```python
from build123d import *

# Parameters (mm, degrees)
EXTRUDE_2_DEPTH          = 51
HOLE_WIZARD_M2_5_1_D     = 2.05
HOLE_WIZARD_M2_5_1_DEPTH = 4.75
HOLE_WIZARD_M2_5_1_TIP   = 0.615882135
SKETCH_7_R               = 11
SKETCH_7_R_2             = 2.5
EXTRUDE_3_DEPTH          = 2
SKETCH_7_2_R             = 2.5
EXTRUDE_4_DEPTH          = 20
SKETCH_8_W               = 15
SKETCH_8_H               = 0.5
CUT_EXTRUDE_1_DEPTH      = 1.5
SKETCH_9_W               = 15.5
SKETCH_9_H               = 2.6
EXTRUDE_5_DEPTH          = 6


with BuildPart() as part:
    # 草图1 → 凸台-拉伸2 (new body)
    with BuildSketch(Plane.XY):
        with BuildLine():
            Line((-12.1, -14.1), (12.1, -14.1))
            ThreePointArc((12.1, -14.1), (13.514213562, -13.514213562), (14.1, -12.1))
            Line((14.1, -12.1), (14.1, 12.1))
            ThreePointArc((14.1, 12.1), (13.514213562, 13.514213562), (12.1, 14.1))
            Line((12.1, 14.1), (-12.1, 14.1))
            ThreePointArc((-12.1, 14.1), (-13.514213562, 13.514213562), (-14.1, 12.1))
            Line((-14.1, 12.1), (-14.1, -12.1))
            ThreePointArc((-14.1, -12.1), (-13.514213562, -13.514213562), (-12.1, -14.1))
        make_face()
    extrude(amount=EXTRUDE_2_DEPTH)

    # M2.5 螺纹孔1
    with Locations(Plane(origin=(0, 0, 0), x_dir=(-1, 0, 0), z_dir=(0, 0, -1))):
        with Locations((-11.5, 11.5), (11.5, 11.5), (11.5, -11.5), (-11.5, -11.5)):
            Hole(HOLE_WIZARD_M2_5_1_D / 2, depth=HOLE_WIZARD_M2_5_1_DEPTH)
            with Locations((0, 0, -(HOLE_WIZARD_M2_5_1_DEPTH + HOLE_WIZARD_M2_5_1_TIP / 2))):  # 118° drill point
                Cone(0, HOLE_WIZARD_M2_5_1_D / 2, HOLE_WIZARD_M2_5_1_TIP, mode=Mode.SUBTRACT)

    # 草图7 → 凸台-拉伸3 (add)
    with BuildSketch(Plane.XY):
        Circle(SKETCH_7_R)
        Circle(SKETCH_7_R_2, mode=Mode.SUBTRACT)
    extrude(amount=-EXTRUDE_3_DEPTH)

    # 草图7<2> → 凸台-拉伸4 (add)
    with BuildSketch(Plane.XY):
        Circle(SKETCH_7_2_R)
    extrude(amount=-EXTRUDE_4_DEPTH)

    # 草图8 → 切除-拉伸1 (cut, symmetric)
    with BuildSketch(Plane(origin=(0, 0, 0), x_dir=(0, 0, -1), z_dir=(1, 0, 0))):
        with Locations((12.5, 2.25)):
            Rectangle(SKETCH_8_W, SKETCH_8_H)
    extrude(amount=CUT_EXTRUDE_1_DEPTH, both=True, mode=Mode.SUBTRACT)

    # 草图9 → 凸台-拉伸5 (add)
    with BuildSketch(Plane.XY.offset(44)):
        with Locations((0, -15.4)):
            Rectangle(SKETCH_9_W, SKETCH_9_H)
    extrude(amount=EXTRUDE_5_DEPTH)


solid = part.part
```
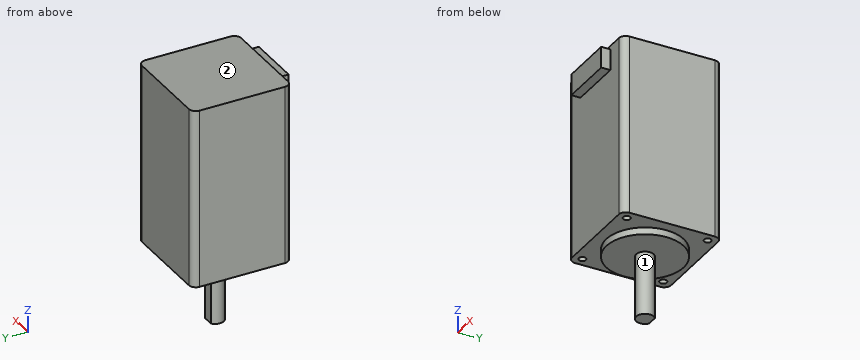
Geometry: final body of the model. Coordinates: model frame, mm. Face numbers are marked on the shaded views. A direction names the side the tool comes from. Coordinates: 2 decimals unless noted, no trailing zeros. Write each loop counter-clockwise with the first axis right and the second up, starting at its lowest first coordinate (ties: lowest second). Pieces come first, ordered by that corner, then holes. Notation, with made-up numbers: M -40,56 L -18,56 A24 ccw -18,90 Z; hole C 55,72 d7. An arc over 180 degrees is marked long. Answer as CSV lines item,"result". Start each with the question number.
Q1. Reachability of the marked faces 1 and 2 from +Z, -Z, +X, -X, +Y, -Y: full face, straight path, thin tool, end or side. Return the list, or none.
Q2. Cut plane B-B on y = 0. Return the cut outline in (x, z).
Q3. Pin query (flat end, axial travel): P1, Ø0.9, axis at x = -0.5, z = -10, coming from the +Y side; P2, Ø5, axis at x = 2.5, z = 14.5, coming from the -Y side; P3, Ø1.8, axis at x = 11.5, y = 11.5, coming from the -Z side. Return the tip coordinate at first contact, or that it passes through.
Q4. Cut plane A-A on z = 4. Return the cut outline in (x, y) (3 decimals).
Q5. Line query: line 1 (Y direction, x = -11.5, z = 2.7) (3 decimals); line 2 (X direction, y = -11, z = 3). Output: solid intervals per line, ascending. Write a range as from..to.
Q6. Cut plane D-D on x = 0. Return the cut outline in (y, z), then the cut area to 3 significant figures.
Q7. Cut plane C-C on z = 45.5. Return the cut outline in (x, y), then the cut area to 3 significant figures.
Findings below:
1,face 1,"-Z"
1,face 2,"+Z, +X, -X, +Y, -Y"
2,outline,"M -14.1,0 L -11,0 L -11,-2 L -2.5,-2 L -2.5,-20 L 2.5,-20 L 2.5,-2 L 11,-2 L 11,0 L 14.1,0 L 14.1,51 L -14.1,51 Z"
3,P1,"stops at y = 2"
3,P2,"stops at y = -14.1"
3,P3,"stops at z = 4.83"
4,outline,"M -14.1,-12.1 A2 ccw -12.1,-14.1 L 12.1,-14.1 A2 ccw 14.1,-12.1 L 14.1,12.1 A2 ccw 12.1,14.1 L -12.1,14.1 A2 ccw -14.1,12.1 Z; hole C -11.5,-11.5 d2.05; hole C -11.5,11.5 d2.05; hole C 11.5,-11.5 d2.05; hole C 11.5,11.5 d2.05"
5,line 1,"y = -14.1..-12.525, -10.475..10.475, 12.525..14.1"
5,line 2,"x = -14.1..-12.39, -10.61..10.61, 12.39..14.1"
6,outline,"M -16.7,44 L -14.1,44 L -14.1,0 L -11,0 L -11,-2 L -2.5,-2 L -2.5,-20 L 2,-20 L 2,-5 L 2.5,-5 L 2.5,-2 L 11,-2 L 11,0 L 14.1,0 L 14.1,51 L -14.1,51 L -14.1,50 L -16.7,50 Z"
6,area,"1,580 mm2"
7,outline,"M -14.1,-12.1 A2 ccw -12.1,-14.1 L -7.75,-14.1 L -7.75,-16.7 L 7.75,-16.7 L 7.75,-14.1 L 12.1,-14.1 A2 ccw 14.1,-12.1 L 14.1,12.1 A2 ccw 12.1,14.1 L -12.1,14.1 A2 ccw -14.1,12.1 Z"
7,area,"832 mm2"
